Build history of the part. All positions in model axes, mm. Round coordinates to 2 decimals unless told otherwise and drop trailing zeros. Write each loop counter-clockwise with the first axis right and the second up, starting at its lowest first coordinate (ties: lowest second). Pieces come first, ordered by that corner, then holes. Notation, with made-up numbers: (19.25, 51) - (56.25, 51) arc R14 ccw to (56.25, 58) - close; hole circle Ø2 at (-36, 62.5). An arc over 180 degrees is marked (long way). Answer as a JSON object with one key per item and string values. Group by question number.
Item 1: Slice it at A-A, the plane x = 0. List the corners of the cut face in (y, z).
Item 2: Probe line 1 (X direction, y = 3.75, z = -1.5); line 2 (Y direction, x = -6, z = 2.75); line 3 (Y direction, x = 0.25, z = -1.25). List the from-to ranges inside material, lowest first. Write a range as from..to.
Item 3: Slice it at C-C, the plane z = -2.75. List the corners of the cut face in (x, y), then the cut area to 3 significant figures.
Item 4: Slice it at D-D, the plane y = 4. List the corners of the cut face in (x, z).
Item 5: Flat gauge pins, fed straight in: pin 1 (3 mm diameter, centred on x = -4.5, z = -1.5, fed in from +Y); pin 2 (4 mm diameter, centred on x = 3, z = -3, fed in from +Y); pin 3 (8 mm diameter, centred on x = 5, y = 4.5, fed in from +Z). Where does each tip first touch, or does it go through?
Item 6: Two-plate mould, pull along X, no slides. Class faces 1 (the flat face through (2, 0, -5)), 2 (the cylindrical face through (7.06, -2.8, -0.94)), 3 (the cylindrical face through (-1.172, 8.923, -0.944)): +X half, -X half, draft (parallel to the pull), parting line (faces both ways), or undercut.
Item 7: Slice it at B-B, the plane y = 0. List the corners of the cut face in (x, z).
Autodesk Inventor part; units mm, degrees
ref_plane "YZ Plane" through (0, 0, 0) normal (1, 0, 0) x (0, 1, 0)
ref_plane "XZ Plane" through (0, 0, 0) normal (0, 1, 0) x (-1, 0, 0)
ref_plane "XY Plane" through (0, 0, 0) normal (0, 0, 1) x (1, 0, 0)
sketch "Sketch1" plane through (0, 0, 0) normal (0, 0, 1) x (1, 0, 0)
  circle A0 centre (0, 0) radius 4
  circle A1 centre (0, 0) radius 9
  point P0 (0, 0)
  dimension "d0" = 18
extrude "Extrusion1" add sketch "Sketch1" along normal blind 3 and the other way blind 5 contours A0 | A1
sketch "Sketch2" plane through (0, 0, 3) normal (0, 0, 1) x (1, 0, 0)
  circle A0 centre (0, 0) radius 6.5 construction
  circle A1 centre (0, 6.5) radius 1.5
  circle A2 centre (-5.6292, 3.25) radius 1.5
  circle A3 centre (-5.6292, -3.25) radius 1.5
  circle A4 centre (0, -6.5) radius 1.5
  circle A5 centre (5.6292, -3.25) radius 1.5
  circle A6 centre (5.6292, 3.25) radius 1.5
  dimension "d5" = 13
  dimension "d6" = 3
  dimension "d9" = 360
extrude "Extrusion2" cut sketch "Sketch2" against normal through all
sketch "Sketch3" plane through (0, 0, 3) normal (0, 0, 1) x (1, 0, 0)
  circle A0 centre (0, 0) radius 1.25
  dimension "d13" = 2.5
extrude "Extrusion3" cut sketch "Sketch3" against normal through all
properties part number "servo shaft flange"
Geometry says:
{
 "1": {"outline": "(-9, -5) - (-8, -5) - (-8, 3) - (-9, 3) - close; (-5, -5) - (-1.25, -5) - (-1.25, 3) - (-5, 3) - close; (1.25, -5) - (5, -5) - (5, 3) - (1.25, 3) - close; (8, -5) - (9, -5) - (9, 3) - (8, 3) - close"},
 "2": {"line 1": "x = -8.18..-7.04, -4.21..4.21, 7.04..8.18", "line 2": "y = -6.71..-4.7, -1.8..1.8, 4.7..6.71", "line 3": "y = -9..-7.98, -5.02..-1.22, 1.22..5.02, 7.98..9"},
 "3": {"outline": "circle Ø18 at (0, 0); hole circle Ø3 at (-5.63, -3.25); hole circle Ø3 at (-5.63, 3.25); hole circle Ø3 at (0, -6.5); hole circle Ø3 at (0, 6.5); hole circle Ø2.5 at (0, 0); hole circle Ø3 at (5.63, -3.25); hole circle Ø3 at (5.63, 3.25)", "area": "207 mm^2"},
 "4": {"outline": "(-8.06, -5) - (-6.93, -5) - (-6.93, 3) - (-8.06, 3) - close; (-4.33, -5) - (4.33, -5) - (4.33, 3) - (-4.33, 3) - close; (6.93, -5) - (8.06, -5) - (8.06, 3) - (6.93, 3) - close"},
 "5": {"pin 1": "stops at y = 8.49", "pin 2": "stops at y = 8.94", "pin 3": "stops at z = 3"},
 "6": {"face 1": "draft", "face 2": "undercut", "face 3": "parting line"},
 "7": {"outline": "(-9, -5) - (-1.25, -5) - (-1.25, 3) - (-9, 3) - close; (1.25, -5) - (9, -5) - (9, 3) - (1.25, 3) - close"}
}
